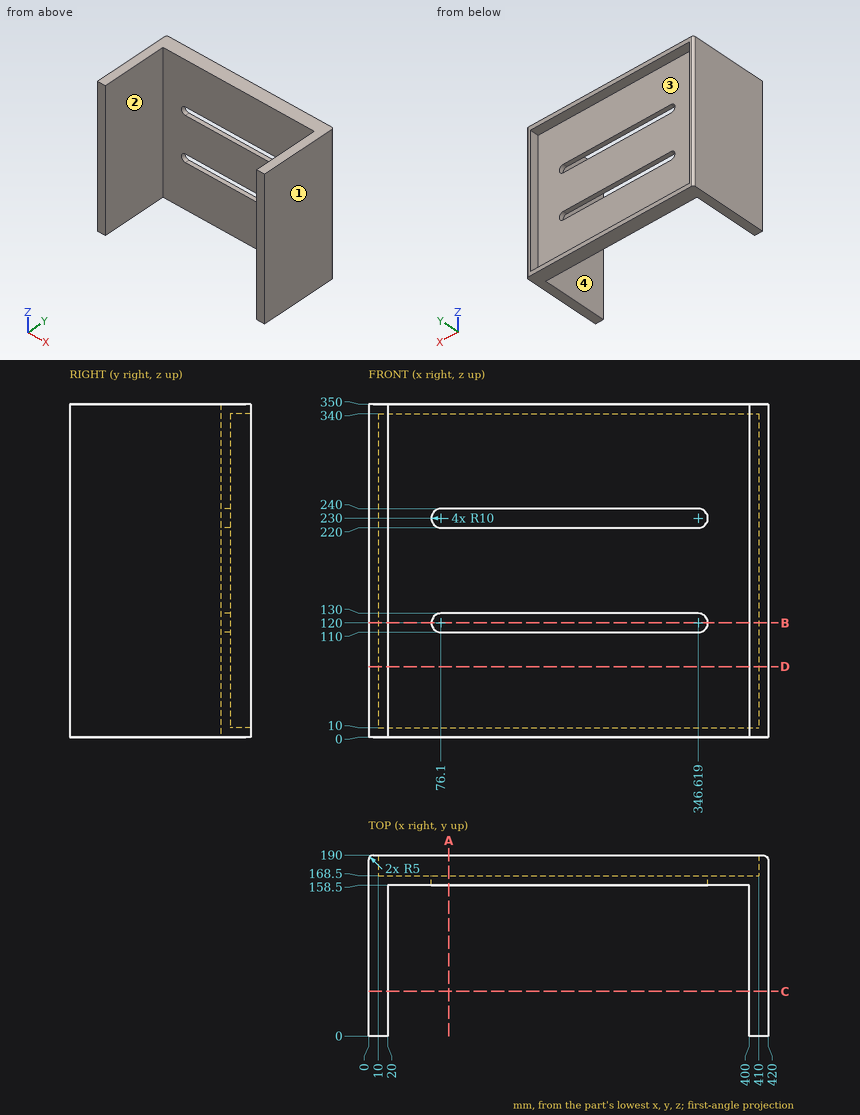
Input: dimensioned drawing with shaded views. Units: mm. Origin: part minimum x, y, z. A direction names the side the tool comes from. Coordinates: 2 decimals unless noted, no trailing zeros. Loops run counter-clockwise (first coordinate to the right, second up) from the corner with the lowest first, then second, coordinate; pieces in that order, holes last. Notation, with made-up numbers: (15.5, 88) -> (37.5, 88) arc R18 ccw to (37.5, 99) -> close; hole circle Ø7 at (64.25, 2.25). An arc over 180 degrees is marked (long way). One line per item, written item: value. Start each with the question number.
Q1. Set-up query: the marked faces 1 and 2. Return all of +Z, -Z, +X, -X, +Y, -Y with unobstructed straight access to the full face (end or side cutting, diameter ignored); none if empty.
Q2. Line query: line 1 along X through (y, z) = (10, 156.5); line 2 along X through (y, z) = (171, 241); line 3 along Y through (x, z) = (345, 314.5). Output: solid intervals per line, ascending.
Q3. Section query B-B, the plane z = 120. Return the cut outline in (x, y), and give its area (3 significant figures).
Q4. Section query C-C, the plane y = 47. Return the cut outline in (x, z), and give its area (3 significant figures).
Q5. Mould query, pull axis Z, two halves, no side actions, for the marked faces 3 and 4. Classes: pulls with the +Z half, pulls with the -Z half, needs draft (parallel to the pull), parting line crosses it, or undercut.
Q6. Contact query for flat-ended pins moving along their axis: P1, Ø3, axis at x = 296, z = 191, coming from the -Y side; P2, Ø1.5, axis at x = 287, z = 180, coming from the +Y side. Output: stop coordinate, or through.
Q7. Section query A-A, the plane x = 84.5. Return the cut outline in (y, z).
Q8. Section query D-D, the plane z = 74. Return the cut outline in (x, y), and give its area (3 significant figures).
Results:
1. face 1: +Z, -Z, +X, +Y, -Y
1. face 2: +Z, -Z, -Y
2. line 1: 0 to 20, 400 to 420
2. line 2: 0 to 10, 410 to 420
2. line 3: 158.5 to 168.5
3. outline: (0, 0) -> (20, 0) -> (20, 158.5) -> (66.1, 158.5) -> (66.1, 168.5) -> (10, 168.5) -> (10, 190) -> (5, 190) arc R5 ccw to (0, 185) -> close; (356.62, 158.5) -> (400, 158.5) -> (400, 0) -> (420, 0) -> (420, 185) arc R5 ccw to (415, 190) -> (410, 190) -> (410, 168.5) -> (356.62, 168.5) -> close
3. area: 8,050 mm^2
4. outline: (0, 0) -> (20, 0) -> (20, 350) -> (0, 350) -> close; (400, 0) -> (420, 0) -> (420, 350) -> (400, 350) -> close
4. area: 14,000 mm^2
5. face 3: undercut
5. face 4: needs draft
6. P1: y = 158.5
6. P2: y = 168.5
7. outline: (158.5, 0) -> (190, 0) -> (190, 10) -> (168.5, 10) -> (168.5, 110) -> (158.5, 110) -> close; (158.5, 130) -> (168.5, 130) -> (168.5, 220) -> (158.5, 220) -> close; (158.5, 240) -> (168.5, 240) -> (168.5, 340) -> (190, 340) -> (190, 350) -> (158.5, 350) -> close
8. outline: (0, 0) -> (20, 0) -> (20, 158.5) -> (400, 158.5) -> (400, 0) -> (420, 0) -> (420, 185) arc R5 ccw to (415, 190) -> (410, 190) -> (410, 168.5) -> (10, 168.5) -> (10, 190) -> (5, 190) arc R5 ccw to (0, 185) -> close
8. area: 11,000 mm^2
